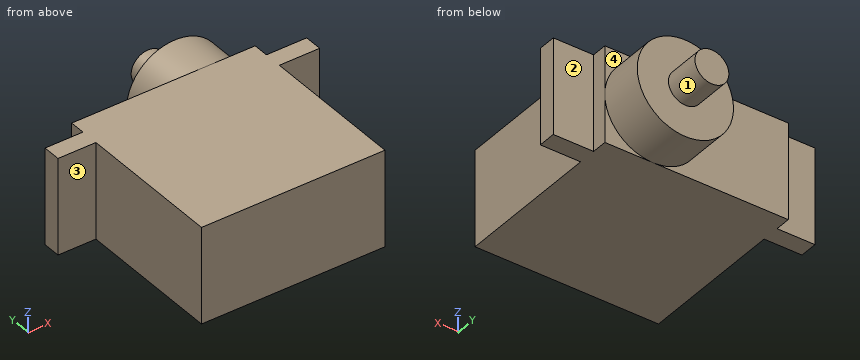
from build123d import *

# Parameters (mm, degrees)
SKETCH1_W           = 22.5
SKETCH1_H           = 11.8
BOSS_EXTRUDE1_DEPTH = 17.9
SKETCH2_W           = 22.5
SKETCH2_H           = 11.8
BOSS_EXTRUDE2_DEPTH = 4.1
SKETCH3_R           = 5.9
BOSS_EXTRUDE3_DEPTH = 5.5
SKETCH4_R           = 2.078257601
BOSS_EXTRUDE4_DEPTH = 4.5
SKETCH5_W           = 32.1
SKETCH5_H           = 11.8
BOSS_EXTRUDE5_DEPTH = 2.2


with BuildPart() as part:
    # Sketch1 → Boss-Extrude1 (new body)
    with BuildSketch(Plane(origin=(0, 0, 0), x_dir=(1, 0, 0), z_dir=(0, 1, 0))):
        with Locations((11.25, 5.9)):
            Rectangle(SKETCH1_W, SKETCH1_H)
    extrude(amount=BOSS_EXTRUDE1_DEPTH)

    # Sketch2 → Boss-Extrude2 (add)
    with BuildSketch(Plane(origin=(0, 17.9, 0), x_dir=(1, 0, 0), z_dir=(0, 1, 0))):
        with Locations((11.25, 5.9)):
            Rectangle(SKETCH2_W, SKETCH2_H)
    extrude(amount=BOSS_EXTRUDE2_DEPTH)

    # Sketch3 → Boss-Extrude3 (add)
    with BuildSketch(Plane(origin=(0, 22, 0), x_dir=(1, 0, 0), z_dir=(0, 1, 0))):
        with Locations((16.6, 5.9)):
            Circle(SKETCH3_R)
    extrude(amount=BOSS_EXTRUDE3_DEPTH)

    # Sketch4 → Boss-Extrude4 (add)
    with BuildSketch(Plane(origin=(0, 27.5, 0), x_dir=(1, 0, 0), z_dir=(0, 1, 0))):
        with Locations((16.6, 5.9)):
            Circle(SKETCH4_R)
    extrude(amount=BOSS_EXTRUDE4_DEPTH)

    # Sketch5 → Boss-Extrude5 (add)
    with BuildSketch(Plane(origin=(0, 17.9, 0), x_dir=(1, 0, 0), z_dir=(0, 1, 0))):
        with Locations((11.4, 5.9)):
            Rectangle(SKETCH5_W, SKETCH5_H)
    extrude(amount=BOSS_EXTRUDE5_DEPTH)


solid = part.part
Here's how the part is built. I have some questions about the finished solid (model axes, mm). Face numbers are marked on the shaded views. A direction names the side the tool comes from. Round coordinates to 2 decimals unless told otherwise and drop trailing zeros. Loops run counter-clockwise (first coordinate to the right, second up) from the corner with the lowest first, then second, coordinate; pieces in that order, holes last. Notation, with made-up numbers: (72, 25.25) - (82, 25.25) arc R16 cw to (82, 29.25) - close; hole circle Ø11 at (83.25, 4). An arc over 180 degrees is marked (long way). One line per question, with ' | ' between items. Start each with the question number.
Q1. Will these pins go through, and if not, where does the flat tip stop? pin 1 (2.5 mm diameter, centred on x = 25, z = -5, fed in from +Y); pin 2 (6 mm diameter, centred on x = 6.5, z = -5, fed in from +Y); pin 3 (6 mm diameter, centred on x = 11, z = -4.5, fed in from -Y); pin 4 (0.6 mm diameter, centred on y = 21, z = -4.5, fed in from -X).
Q2. Please list where these lines run through material, in increasing order: line 1 (X direction, y = 2, z = -4.5); line 2 (Y direction, x = 23, z = -5.5); line 3 (Y direction, x = 16, z = -10). Write a range as [from, to].
Q3. I want a section at A-A (z = -11). Write out the boundary of the cut face in (x, y).
Q4. I want a section at C-C (y = 13). Write out the boundary of the cut face in (x, z).
Q5. I want a section at B-B (x = 15). Write out the boundary of the cut face in (y, z).
Q6. I want a section at D-D (z = -2.5). Write out the boundary of the cut face in (x, y).
Q7. For the marked faces 1, 2, 3 and 4, which set-ups out of +Z, -Z, +X, -X, +Y, -Y let a thin tool reach every point of the face, with its end or its side?
Response values:
1) pin 1: stops at y = 20.1 | pin 2: stops at y = 22 | pin 3: stops at y = 0 | pin 4: stops at x = 0
2) line 1: x = [0, 22.5] | line 2: y = [17.9, 20.1] | line 3: y = [0, 27.5]
3) outline: (-4.65, 17.9) - (0, 17.9) - (0, 0) - (22.5, 0) - (22.5, 17.9) - (27.45, 17.9) - (27.45, 20.1) - (22.5, 20.1) - (22.5, 22) - (19.57, 22) - (19.57, 27.5) - (13.63, 27.5) - (13.63, 22) - (0, 22) - (0, 20.1) - (-4.65, 20.1) - close
4) outline: (0, -11.8) - (22.5, -11.8) - (22.5, 0) - (0, 0) - close
5) outline: (0, -11.8) - (22, -11.8) - (22, -11.58) - (27.5, -11.58) - (27.5, -7.23) - (32, -7.23) - (32, -4.57) - (27.5, -4.57) - (27.5, -0.22) - (22, -0.22) - (22, 0) - (0, 0) - close
6) outline: (-4.65, 17.9) - (0, 17.9) - (0, 0) - (22.5, 0) - (22.5, 17.9) - (27.45, 17.9) - (27.45, 20.1) - (22.5, 20.1) - (22.5, 22) - (21.42, 22) - (21.42, 27.5) - (11.78, 27.5) - (11.78, 22) - (0, 22) - (0, 20.1) - (-4.65, 20.1) - close
7) face 1: +Y | face 2: +Z, -Z, +X, +Y | face 3: +Z, -Z, -X, -Y | face 4: +Z, +X, +Y
